Could you check a few things on this model? Use its own coordinates, in mm. Give positions to 0.01 mm unless a question says otherwise; leave off trailing zeros. Write each loop counter-clockwise with the first axis right and the second up, starting at its lowest first coordinate (ties: lowest second). Pieces come first, ordered by that corner, then holes. Notation, with made-up numbers: M 18.5,64 L 43.5,64 A9 ccw 43.5,69 Z; hole C 89,-31 d2. An arc over 180 degrees is marked long. Answer as a JSON object with one key per item and string values. Group by question number.
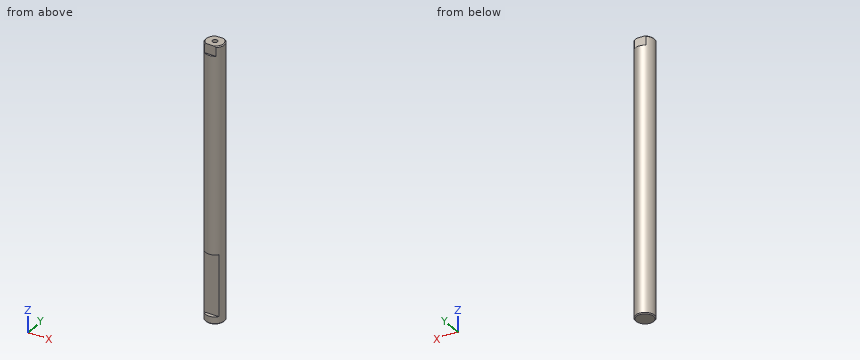
```python
from build123d import *

# Parameters (mm, degrees)
SKETCH1_R                  = 15.875
BOSS_EXTRUDE1_DEPTH        = 228.6
SKETCH2_W                  = 50.8
SKETCH2_H                  = 101.981
CUT_EXTRUDE2_DEPTH         = 9.525
CHAMFER1_SIZE              = 1.5875
SKETCH3_W                  = 19.05
SKETCH3_H                  = 10.048588851
SKETCH3_H_2                = 8.582335087
CUT_EXTRUDE3_DEPTH         = 15.875
M10X1_5_TAPPED_HOLE1_D     = 8.5
M10X1_5_TAPPED_HOLE1_DEPTH = 27.686
M10X1_5_TAPPED_HOLE1_TIP   = 2.553657631


with BuildPart() as part:
    # Sketch1 → Boss-Extrude1 (new body, symmetric)
    with BuildSketch(Plane.XY):
        Circle(SKETCH1_R)
    extrude(amount=BOSS_EXTRUDE1_DEPTH, both=True)

    # Sketch2 → Cut-Extrude2 (cut)
    with BuildSketch(Plane(origin=(0, -19.05, 0), x_dir=(1, 0, 0), z_dir=(0, 1, 0))):
        with Locations((0, 165.1635)):
            Rectangle(SKETCH2_W, SKETCH2_H)
    extrude(amount=CUT_EXTRUDE2_DEPTH, mode=Mode.SUBTRACT)

    # Chamfer1
    chamfer1_edges = [part.edges().sort_by_distance(p)[0] for p in [
        (-15.875, 0, -228.6),
        (-15.875, 0, 228.6),
    ]]
    chamfer(chamfer1_edges, length=CHAMFER1_SIZE)

    # Sketch3 → Cut-Extrude3 (cut)
    with BuildSketch(Plane.XY.offset(228.6)):
        with Locations((0, 17.724294426)):
            Rectangle(SKETCH3_W, SKETCH3_H)
        with Locations((0, -16.991167544)):
            Rectangle(SKETCH3_W, SKETCH3_H_2)
    extrude(amount=-CUT_EXTRUDE3_DEPTH, mode=Mode.SUBTRACT)

    # M10x1.5 Tapped Hole1
    with Locations(Plane.XY.offset(228.6)):
        with Locations((0, 0)):
            Hole(M10X1_5_TAPPED_HOLE1_D / 2, depth=M10X1_5_TAPPED_HOLE1_DEPTH)
            with Locations((0, 0, -(M10X1_5_TAPPED_HOLE1_DEPTH + M10X1_5_TAPPED_HOLE1_TIP / 2))):  # 118° drill point
                Cone(0, M10X1_5_TAPPED_HOLE1_D / 2, M10X1_5_TAPPED_HOLE1_TIP, mode=Mode.SUBTRACT)


solid = part.part
```
1) If we section it at A-A, the plane z = -172: List the corners of the cut face in (x, y) for me (3 decimals), plus the area to 3 significant figures.
2) Please list where these lines run through material, in increasing order: line 1 along Z through (x, y) = (3.5, -10.5); line 2 along Y through (x, z) = (0, 208) (3 decimals); line 3 along Y through (x, z) = (0, 213). Write a range as from..to.
3) I'm going to push flat-ended pins straight in: pin 1 (2 mm diameter, centred on x = -7, z = -81, fed in from +Y); pin 2 (1.6 mm diameter, centred on x = 0, y = 14.5, fed in from +Z) (3 decimals); pin 3 (4 mm diameter, centred on x = -10, z = -35.5, fed in from +Y). Where does each tip first touch, or does it pass through?
4) If we section it at B-B, the plane z = 86.5: List the corners of the cut face in (x, y) for me (3 decimals), plus the area to 3 significant figures.
Taken from the geometry:
{
 "1": {"outline": "M -12.7,-9.525 L 12.7,-9.525 A15.875 ccw long Z", "area": "679 mm²"},
 "2": {"line 1": "-228.6..-216.15, -114.17..228.6", "line 2": "-15.875..-4.25, 4.25..15.875", "line 3": "-12.7..-4.25, 4.25..12.7"},
 "3": {"pin 1": "y = 14.7", "pin 2": "z = 212.725", "pin 3": "y = 13.71"},
 "4": {"outline": "C 0,0 d31.75", "area": "792 mm²"}
}
